Verification items for the finished model (mm, model axes). Coordinates: 2 decimals unless noted, no trailing zeros. Order: outer loops, then holes, each group sorted by start corner. A loop starts at its lowest first (then second) coordinate and runs counter-clockwise, first axis right, second up.
Q1. Cross-section at C-C, the plane z = -9.5. Record the boundary of the cut face in (x, y), and give its area (3 significant figures).
Q2. Cross-section at B-B, the plane z = -4.75. Record the boundary of the cut face in (x, y), and give its area (3 significant figures).
Q3. Cross-section at A-A, the plane x = 0. Record the boundary of the cut face in (y, z), and give its area (3 significant figures).
Q4. Cross-section at D-D, the plane y = 1.75. Record the boundary of the cut face in (x, z).
Q5. Depth check by flat-ended pin: P1, Ø2, axis at x = -5.5, z = 8.5, coming from the +Y side; P2, Ø5.5, axis at x = 0, z = 0, coming from the -Y side; P3, Ø1.5, axis at y = 2, z = -8, coming from the +X side; P4, Ø1.5, axis at y = 5, z = 7.5, coming from the -X side. Enter the tip coordinate at first touch or a pass-through.
Q6. Thickness scan on line 1 (X direction, y = 2, z = -4.75); line 2 (Z direction, x = -8.5, y = 1.25); line 3 (Z direction, x = 0.75, y = 1.75). Record the ranges inside material, lowest first.
Q7. Draft check along Z on faces 1 (the cylindrical face through (1.802, 7.071, 5.723)), 2 (the flat face through (3, 5, 5.5)), 3 (the cylindrical face through (0.05, 2.54, 8.3)), 4 (the cylindrical face through (0.05, 2.54, -10.7)). Enter one of: pulls with the +Z half, pulls with the -Z half, needs draft (parallel to the pull), parting line crosses it, or undercut.
from build123d import *

# Parameters (mm, degrees)
SKETCH1_R           = 12.7
SKETCH1_R_2         = 3
BOSS_EXTRUDE1_DEPTH = 5
SKETCH2_R           = 6
SKETCH2_R_2         = 3
BOSS_EXTRUDE2_DEPTH = 4.2
SKETCH3_R           = 1.2
CUT_EXTRUDE1_DEPTH  = 19.643497526


with BuildPart() as part:
    # Sketch1 → Boss-Extrude1 (new body)
    with BuildSketch(Plane(origin=(0, 0, 0), x_dir=(1, 0, 0), z_dir=(0, 1, 0))):
        with Locations(Location((0, 0, 0), (0, 0, 270))):
            Circle(SKETCH1_R)
        with Locations(Location((0, 0, 0), (0, 0, 270))):
            Circle(SKETCH1_R_2, mode=Mode.SUBTRACT)
    extrude(amount=BOSS_EXTRUDE1_DEPTH)

    # Sketch2 → Boss-Extrude2 (add)
    with BuildSketch(Plane(origin=(0, 5, 0), x_dir=(1, 0, 0), z_dir=(0, 1, 0))):
        with Locations(Location((0, 0, 0), (0, 0, 270))):
            Circle(SKETCH2_R)
        with Locations(Location((0, 0, 0), (0, 0, 270))):
            Circle(SKETCH2_R_2, mode=Mode.SUBTRACT)
    extrude(amount=BOSS_EXTRUDE2_DEPTH)

    # Sketch3 → Cut-Extrude1 (cut, through all)
    with BuildSketch(Plane(origin=(0, 5, 0), x_dir=(1, 0, 0), z_dir=(0, 1, 0))):
        with Locations(Location((0, 9.5, 0), (0, 0, 270))):
            Circle(SKETCH3_R)
        with Locations(Location((8.227241336, 4.75, 0), (0, 0, 270))):
            Circle(SKETCH3_R)
        with Locations(Location((8.227241336, -4.75, 0), (0, 0, 270))):
            Circle(SKETCH3_R)
        with Locations(Location((0, -9.5, 0), (0, 0, 270))):
            Circle(SKETCH3_R)
        with Locations(Location((-8.227241336, -4.75, 0), (0, 0, 270))):
            Circle(SKETCH3_R)
        with Locations(Location((-8.227241336, 4.75, 0), (0, 0, 270))):
            Circle(SKETCH3_R)
    extrude(amount=-CUT_EXTRUDE1_DEPTH, mode=Mode.SUBTRACT)


solid = part.part
Check values:
1. outline: (-8.43, 0) - (-1.2, 0) - (-1.2, 5) - (-8.43, 5) - close; (1.2, 0) - (8.43, 0) - (8.43, 5) - (1.2, 5) - close
1. area: 72.3 mm2
2. outline: (-11.78, 0) - (-9.43, 0) - (-9.43, 5) - (-11.78, 5) - close; (-7.03, 0) - (7.03, 0) - (7.03, 5) - (3.67, 5) - (3.67, 9.2) - (-3.67, 9.2) - (-3.67, 5) - (-7.03, 5) - close; (9.43, 0) - (11.78, 0) - (11.78, 5) - (9.43, 5) - close
2. area: 125 mm2
3. outline: (0, -12.7) - (5, -12.7) - (5, -10.7) - (0, -10.7) - close; (0, -8.3) - (5, -8.3) - (5, -6) - (9.2, -6) - (9.2, -3) - (0, -3) - close; (0, 3) - (9.2, 3) - (9.2, 6) - (5, 6) - (5, 8.3) - (0, 8.3) - close; (0, 10.7) - (5, 10.7) - (5, 12.7) - (0, 12.7) - close
3. area: 98.2 mm2
4. outline: circle Ø25.4 at (0, 0); hole circle Ø2.4 at (-8.23, -4.75); hole circle Ø2.4 at (-8.23, 4.75); hole circle Ø6 at (0, 0); hole circle Ø2.4 at (0, -9.5); hole circle Ø2.4 at (0, 9.5); hole circle Ø2.4 at (8.23, -4.75); hole circle Ø2.4 at (8.23, 4.75)
5. P1: stops at y = 5
5. P2: passes through
5. P3: stops at x = 10.43
5. P4: stops at x = -10.76
6. line 1: x = -11.78 to -9.43, -7.03 to 7.03, 9.43 to 11.78
6. line 2: z = -9.44 to -5.92, -3.58 to 3.58, 5.92 to 9.44
6. line 3: z = -12.68 to -10.44, -8.56 to -2.9, 2.9 to 8.56, 10.44 to 12.68
7. face 1: parting line crosses it
7. face 2: needs draft
7. face 3: undercut
7. face 4: undercut
